Geometry check sheet. Reference: the model listing, model coordinates, mm. A direction names the side the tool comes from. Round coordinates to 2 decimals unless told otherwise and drop trailing zeros. Order: outer loops, then holes, each group sorted by start corner. A loop starts at its lowest first (then second) coordinate and runs counter-clockwise, first axis right, second up.
```python
from build123d import *

# Parameters (mm, degrees)
SKETCH1_R               = 35
BOSS_EXTRUDE1_DEPTH     = 10
SKETCH27_W              = 8.45046724
SKETCH27_H              = 8.572937779
CUT_EXTRUDE8_DEPTH      = 51.497524692
CUT_EXTRUDE9_DEPTH      = 51.497524692
CUT_EXTRUDE9_DEPTH_BACK = 51.497524692
SKETCH34_R              = 2
SKETCH35_R              = 2
CUT_EXTRUDE10_DEPTH     = 51.497524692
SKETCH36_R              = 2
CUT_EXTRUDE11_DEPTH     = 51.497524692
SKETCH37_R              = 2
CUT_EXTRUDE12_DEPTH     = 51.497524692
SKETCH39_R              = 32
CUT_EXTRUDE14_DEPTH     = 3
SKETCH40_R              = 1.6
CUT_EXTRUDE16_DEPTH     = 35
SKETCH49_W              = 3
SKETCH49_H              = 26.802326962
CUT_EXTRUDE18_DEPTH     = 51.49752485


with BuildPart() as part:
    # Sketch1 → Boss-Extrude1 (new body)
    with BuildSketch(Plane(origin=(0, 0, 0), x_dir=(1, 0, 0), z_dir=(0, 1, 0))):
        with Locations(Location((0, 0, 0), (0, 0, 270))):
            Circle(SKETCH1_R)
    extrude(amount=BOSS_EXTRUDE1_DEPTH)

    # Sketch27 → Cut-Extrude8 (cut, through all)
    with BuildSketch(Plane(origin=(0, 10, 0), x_dir=(1, 0, 0), z_dir=(0, 1, 0))):
        with Locations((31.027560582, -0.794372815)):
            Rectangle(SKETCH27_W, SKETCH27_H)
    extrude(amount=-CUT_EXTRUDE8_DEPTH, mode=Mode.SUBTRACT)

    # Sketch34 → Cut-Extrude9 (cut, two sides: drawn at the far end of the back side and taken through both)
    with BuildSketch(Plane(origin=(0, 10, 0), x_dir=(1, 0, 0), z_dir=(0, 1, 0)).offset(-CUT_EXTRUDE9_DEPTH_BACK)):
        with Locations(Location((-17, 17, 0), (0, 0, 270))):
            Circle(SKETCH34_R)
    extrude(amount=CUT_EXTRUDE9_DEPTH + CUT_EXTRUDE9_DEPTH_BACK, mode=Mode.SUBTRACT)

    # Sketch35 → Cut-Extrude10 (cut, through all)
    with BuildSketch(Plane(origin=(0, 0, 0), x_dir=(-1, 0, 0), z_dir=(0, -1, 0))):
        with Locations(Location((-17, 17, 0), (0, 0, 90))):
            Circle(SKETCH35_R)
    extrude(amount=-CUT_EXTRUDE10_DEPTH, mode=Mode.SUBTRACT)

    # Sketch36 → Cut-Extrude11 (cut, through all)
    with BuildSketch(Plane(origin=(0, 0, 0), x_dir=(-1, 0, 0), z_dir=(0, -1, 0))):
        with Locations(Location((17, -17, 0), (0, 0, 90))):
            Circle(SKETCH36_R)
    extrude(amount=-CUT_EXTRUDE11_DEPTH, mode=Mode.SUBTRACT)

    # Sketch37 → Cut-Extrude12 (cut, through all)
    with BuildSketch(Plane.XZ):
        with Locations(Location((17, 17, 0), (0, 0, 270))):
            Circle(SKETCH37_R)
    extrude(amount=-CUT_EXTRUDE12_DEPTH, mode=Mode.SUBTRACT)

    # Sketch39 → Cut-Extrude14 (cut)
    with BuildSketch(Plane(origin=(0, 10, 0), x_dir=(1, 0, 0), z_dir=(0, 1, 0))):
        Circle(SKETCH39_R)
    extrude(amount=-CUT_EXTRUDE14_DEPTH, mode=Mode.SUBTRACT)

    # Sketch40 → Cut-Extrude16 (cut)
    with BuildSketch(Plane(origin=(26.802326962, 0, 0), x_dir=(0, 0, -1), z_dir=(1, 0, 0))):
        with Locations((-0.847360281, 3.801055622)):
            Circle(SKETCH40_R)
    extrude(amount=-CUT_EXTRUDE16_DEPTH, mode=Mode.SUBTRACT)

    # Sketch49 → Ø6.0mm Dowel Hole6 (revolve, cut)
    with BuildSketch(Plane(origin=(-8.197673038, 3.801055622, 0.847360281), x_dir=(0, 0, -1), z_dir=(0, 1, 0))):
        with Locations((1.5, 13.401163481)):
            Rectangle(SKETCH49_W, SKETCH49_H)
    revolve(axis=Axis((-1.847673038, 3.801055622, 0.847360281), (-1, 0, 0)), mode=Mode.SUBTRACT)

    # Sketch52 → Cut-Extrude18 (cut, through all)
    with BuildSketch(Plane(origin=(0, 0, 0), x_dir=(-1, 0, 0), z_dir=(0, -1, 0))):
        Polygon((-26.802326962, 3.492096074), (-1.999842463, 3.492096074), (-1.999842463, 10.092096074), (-33.513424129, 10.092096074), (-39.471976124, 10.092096074), (-42.019310815, 10.092096074), (-42.019310815, 3.492096074), align=None)
    extrude(amount=-CUT_EXTRUDE18_DEPTH, mode=Mode.SUBTRACT)


solid = part.part
```
(1) Sectioned sample at C-C, the plane z = -23.5. Record the cut outline in (x, y).
Returned:
outline: (-25.94, 0) - (25.94, 0) - (25.94, 10) - (21.72, 10) - (21.72, 7) - (-21.72, 7) - (-21.72, 10) - (-25.94, 10) - close
(2) Sectioned sample at D-D, the plane z = 17. Record the cut outline in (x, y), and give its area (3 significant figures).
Returned:
outline: (-30.59, 0) - (-19, 0) - (-19, 7) - (-27.11, 7) - (-27.11, 10) - (-30.59, 10) - close; (-15, 0) - (15, 0) - (15, 7) - (-15, 7) - close; (19, 0) - (30.59, 0) - (30.59, 10) - (27.11, 10) - (27.11, 7) - (19, 7) - close
area: 393 mm2
(3) Set-up check for faces 5 (the flat face through (-8.198, 5.1, 2.1)), 6 (the cylindrical face through (-15, 3, 17)), 7 (the flat face through (26.802, 2, 1)), 8 (the cylindrical face through (-31.974, 8.521, 1.282)): record each of +Z, -Z, +X, -X, +Y, -Y from which the full face is reachable in a straight line by a thin tool's end or side.
Returned:
face 5: -X
face 6: +Y, -Y
face 7: +X, +Y, -Y
face 8: +Y
(4) Draft check along Y on faces 1 (the flat face through (0, 0, 0)), 2 (the flat face through (31, 4, 5.081)), 3 (the cylindrical face through (-21.79, 6.73, 1.5)), 4 (the flat face through (-1, 7, 0)). Enter one of: released by +Y, released by -Y, zero draft, split by the parting line, or undercut.
Returned:
face 1: released by -Y
face 2: zero draft
face 3: undercut
face 4: released by +Y
(5) Sectioned sample at B-B, the plane x = -17. Record the cut outline in (y, z), and give its area (3 significant figures).
Returned:
outline: (0, -30.59) - (10, -30.59) - (10, -27.11) - (7, -27.11) - (7, -19) - (0, -19) - close; (0, -15) - (7, -15) - (7, 15) - (0, 15) - close; (0, 19) - (7, 19) - (7, 27.11) - (10, 27.11) - (10, 30.59) - (0, 30.59) - close; hole circle Ø6 at (3.8, 0.85)
area: 365 mm2
(6) Material ranges on line 1 (X direction, y = 3, z = -17); line 2 (X direction, y = 7.95, z = 0); line 3 (Y direction, x = 1, z = -2), recorded low to high.
Returned:
line 1: x = -30.59 to -19, -15 to 15, 19 to 30.59
line 2: x = -35 to -32
line 3: y = 0 to 7
(7) Sectioned sample at A-A, the plane x = 11. Record the cut outline in (y, z), and give its area (3 significant figures).
Returned:
outline: (0, -33.23) - (10, -33.23) - (10, -30.05) - (7, -30.05) - (7, -10.09) - (0, -10.09) - close; (0, -3.49) - (7, -3.49) - (7, 30.05) - (10, 30.05) - (10, 33.23) - (0, 33.23) - close; hole circle Ø3.2 at (3.8, 0.85)
area: 430 mm2
(8) Depth check by flat-ended pin: P1, Ø1, axis at x = 23.5, y = 1.5, coming from the -Z side; P2, Ø1, axis at x = 18.5, y = 2, coming from the +Z side; P3, Ø6.5, axis at x = -17, z = -17, coming from the +Y side. Enter the tip coordinate at first touch or a pass-through.
Returned:
P1: stops at z = -26.38
P2: stops at z = 30.02
P3: stops at y = 7
